CAD build for the part. Positions are in the model's coordinates, mm. Round coordinates to 2 decimals unless told otherwise and drop trailing zeros. Loops run counter-clockwise (first coordinate to the right, second up) from the corner with the lowest first, then second, coordinate; pieces in that order, holes last.
from build123d import *

# Parameters (mm, degrees)
SKETCH1_R = 20
PCB_DEPTH = 0.8


with BuildPart() as part:
    # Sketch1 → PCB (new body)
    with BuildSketch(Plane(origin=(0, 0, 0), x_dir=(1, 0, 0), z_dir=(0, 1, 0))):
        with Locations(Location((0, 0, 0), (0, 0, 270))):
            Circle(SKETCH1_R)
    extrude(amount=PCB_DEPTH)

    # Sketch3 → Revolve1 (revolve)
    with BuildSketch(Plane(origin=(0, 0, 0), x_dir=(0, 0, -1), z_dir=(1, 0, 0)), mode=Mode.PRIVATE) as revolve1_sk:
        with BuildLine():
            Line((-16.835, 7.13), (-16.835, 0.8))
            Line((-16.835, 0.8), (-19.526653767, 0.8))
            Line((-19.526653767, 0.8), (-19.526653767, 2.3))
            ThreePointArc((-19.526653767, 2.3), (-19.599683526, 5.505697894), (-16.835, 7.13))
        make_face()
    revolve1 = revolve(revolve1_sk.sketch.rotate(Axis((0, 7.13, 16.835), (0, -1, 0)), 180), axis=Axis((0, 7.13, 16.835), (0, -1, 0)))

    # Mirror1: Revolve1 across plane
    add(revolve1.mirror(Plane.XY))


solid = part.part
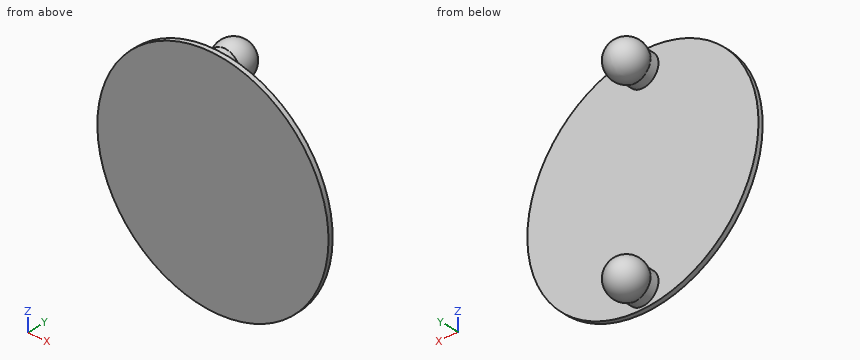
Item 1: Wall check: L1, parallel to Y at x = -4, z = -2.5; L2, parallel to X at y = 5.5, z = -17.5; L3, parallel to Z at x = 2, y = 5.5. Give the ranges that are in metal, low to high.
Verdict:
L1: y = 0 to 0.8
L2: x = -2.69 to 2.69
L3: z = -18.75 to -14.92, 14.92 to 18.75
Item 2: Flat gauge pins, fed straight in: P1, Ø10, axis at x = -1.5, z = -8, coming from the +Y side; P2, Ø1.5, axis at y = 1.5, z = -4, coming from the -X side. Where does each tip first touch, or does it go through?
Verdict:
P1: stops at y = 0.8
P2: stops at x = -19.65
Item 3: Cut at C-C (z = 0). List the corners of the cut face in (x, y).
Verdict:
outline: (-20, 0) - (20, 0) - (20, 0.8) - (-20, 0.8) - close
Item 4: Cut at B-B (z = 12). List the corners of the cut face in (x, y), plus the area to 3 significant figures.
Verdict:
outline: (-16, 0) - (16, 0) - (16, 0.8) - (-16, 0.8) - close
area: 25.6 mm2
Item 5: Cut at A-A (x = 0). List the corners of the cut face in (y, z) (3 decimals), plus the area to 3 significant figures.
Verdict:
outline: (0, -20) - (0.8, -20) - (0.8, -19.527) - (2.3, -19.527) arc R3.165 ccw (long way) to (2.3, -14.143) - (0.8, -14.143) - (0.8, 14.143) - (2.3, 14.143) arc R3.165 ccw (long way) to (2.3, 19.527) - (0.8, 19.527) - (0.8, 20) - (0, 20) - close
area: 99.7 mm2
